```python
from build123d import *

# Parameters (mm, degrees)
CROQUIS1_W              = 250
CROQUIS1_H              = 220
SALIENTE_EXTRUIR1_DEPTH = 3.175
REDONDEO1_R             = 60
CROQUIS2_R              = 6.35
CORTAR_EXTRUIR1_DEPTH   = 6.35


with BuildPart() as part:
    # Croquis1 → Saliente-Extruir1 (new body)
    with BuildSketch(Plane.XY):
        with Locations((125, 110)):
            Rectangle(CROQUIS1_W, CROQUIS1_H)
    extrude(amount=SALIENTE_EXTRUIR1_DEPTH)

    # Redondeo1
    redondeo1_edges = [part.edges().sort_by_distance(p)[0] for p in [
        (250, 0, 1.5875),
        (0, 0, 1.5875),
    ]]
    fillet(redondeo1_edges, radius=REDONDEO1_R)

    # Croquis2 → Cortar-Extruir1 (cut)
    with BuildSketch(Plane.XY.offset(3.175)):
        with Locations((125, 60)):
            Circle(CROQUIS2_R)
    extrude(amount=-CORTAR_EXTRUIR1_DEPTH, mode=Mode.SUBTRACT)


solid = part.part
```
The listing builds one solid part. Answer for the finished solid, in the listing's coordinates (mm). Give positions to 0.01 mm unless a question says otherwise; leave off trailing zeros. Order: outer loops, then holes, each group sorted by start corner. A loop starts at its lowest first (then second) coordinate and runs counter-clockwise, first axis right, second up. Notation, with made-up numbers: (22.5, -6) - (52.5, -6) arc R11 ccw to (52.5, 9) - close; hole circle Ø1 at (47, -19). An arc over 180 degrees is marked (long way). Use one line per item in the form item = value. Start each with the question number.
(1) The mould has two halves that part along Y. Classify faces 1 (the cylindrical face through (17.11, 18.04, 1.61)), 2 (the cylindrical face through (130.866, 57.568, 1.61)), 3 (the flat face through (123, 112, 3.175)): released by +Y, released by -Y, zero draft, split by the parting line, or undercut.
(2) A flat-ended cylindrical pin translates along its axis: pin 1 Ø1.5 at (y, z) = (34, 2) entering from -X. Find the tip coordinate at first contact, or state that the pin passes through.
(3) A cutting plane is placed at A-A, the plane x = 125. Write down the section's boundary in (y, z) (3 decimals), then the cut area to 3 significant figures.
(4) Consider line 1 (Y direction, x = 125, z = 2.3); line 2 (X direction, y = 64, z = 1.2); line 3 (Y direction, x = 212, z = 2.95). Determine where each line is inside the solid, lowest interval first. Write a range as from..to.
(5) A cutting plane is placed at C-C, the plane y = 17.5. Write down the section's boundary in (x, z) (3 decimals).
(6) A cutting plane is placed at D-D, the plane x = 233. Write down the section's boundary in (y, z) (3 decimals).
(7) A cutting plane is placed at B-B, the plane z = 1.7. Write down the section's boundary in (x, y).
Ans:
q1.face_1 = released by -Y
q1.face_2 = undercut
q1.face_3 = zero draft
q2.pin_1 = 5.57
q3.outline = (0, 0) - (53.65, 0) - (53.65, 3.175) - (0, 3.175) - close; (66.35, 0) - (220, 0) - (220, 3.175) - (66.35, 3.175) - close
q3.area = 658 mm^2
q4.line_1 = 0..53.65, 66.35..220
q4.line_2 = 0..120.07, 129.93..250
q4.line_3 = 4.18..220
q5.outline = (17.647, 0) - (232.353, 0) - (232.353, 3.175) - (17.647, 3.175) - close
q6.outline = (18.155, 0) - (220, 0) - (220, 3.175) - (18.155, 3.175) - close
q7.outline = (0, 60) arc R60 ccw to (60, 0) - (190, 0) arc R60 ccw to (250, 60) - (250, 220) - (0, 220) - close; hole circle Ø12.7 at (125, 60)
